For this review, take the finished solid that the model builds, in its own axes (mm). A direction names the side the tool comes from. Coordinates: 2 decimals unless noted, no trailing zeros. Write each loop counter-clockwise with the first axis right and the second up, starting at its lowest first coordinate (ties: lowest second). Pieces come first, ordered by that corner, then holes.
```python
from build123d import *

# Parameters (mm, degrees)
SKETCH8_W            = 52.5
SKETCH8_H            = 15.75
SKETCH8_R            = 0.6
SKETCH8_W_2          = 15.75
SKETCH8_H_2          = 6
BOSS_EXTRUDE13_DEPTH = 1.5


with BuildPart() as part:
    # Sketch8 → Boss-Extrude13 (new body)
    with BuildSketch(Plane.ZY):
        with Locations((-25.5, 6.625)):
            Rectangle(SKETCH8_W, SKETCH8_H)
        with Locations((-49.5, 4.75)):
            Circle(SKETCH8_R, mode=Mode.SUBTRACT)
        with Locations((-1.5, 4.75)):
            Circle(SKETCH8_R, mode=Mode.SUBTRACT)
        with Locations((-28.375, 5.75)):
            Rectangle(SKETCH8_W_2, SKETCH8_H_2, mode=Mode.SUBTRACT)
    extrude(amount=BOSS_EXTRUDE13_DEPTH)


solid = part.part
```
1) Consider section C-C (x = -0.55). Give the boundary of the cut face in (y, z).
2) The part is to be moulded in two halves that separate along Z. For faces 1 (the face through (-1, 7, -51.75)), 2 (the face through (-1, -1.25, -26)), 3 (the face through (-0.74, 4.164, -1.63)), say which applies: pulls with the +Z half, pulls with the -Z half, needs draft (parallel to the pull), parting line crosses it, or undercut.
3) Consider section B-B (y = 7.5). Give the boundary of the cut face in (x, z).
4) Clearance check with a flat-ended pin moving along its axis: P1, Ø0.7, axis at y = 4.75, z = -1.5, coming from the +X side. State where the tip first meets the part, or that it passes through.
5) Consider section A-A (z = -21.5). Give the boundary of the cut face in (x, y), then the cut area to 3 significant figures.
6) Tool access review of faces 4 (the face through (-1, 6, -20.5)), 5 (the face through (-1.5, 10, -26)): name each direction out of +Z, -Z, +X, -X, +Y, -Y from which nothing blocks a thin tool from reaching the whole face with its end or side.
7) Consider section D-D (y = 4.75). Give the boundary of the cut face in (x, z), then the cut area to 3 significant figures.
8) For L1, parallel to Y at x = -0.4, z = -49.5; L2, parallel to Z at x = -0.2, y = 6, list the stretches that pass through material, from the lowest coordinate up.
Results:
1. outline: (-1.25, -51.75) - (14.5, -51.75) - (14.5, 0.75) - (-1.25, 0.75) - close; hole (2.75, -36.25) - (8.75, -36.25) - (8.75, -20.5) - (2.75, -20.5) - close; hole circle Ø1.2 at (4.75, -49.5); hole circle Ø1.2 at (4.75, -1.5)
2. face 1: pulls with the -Z half
2. face 2: needs draft
2. face 3: undercut
3. outline: (-1.5, -51.75) - (0, -51.75) - (0, -36.25) - (-1.5, -36.25) - close; (-1.5, -20.5) - (0, -20.5) - (0, 0.75) - (-1.5, 0.75) - close
4. P1: passes through
5. outline: (-1.5, -1.25) - (0, -1.25) - (0, 2.75) - (-1.5, 2.75) - close; (-1.5, 8.75) - (0, 8.75) - (0, 14.5) - (-1.5, 14.5) - close
5. area: 14.6 mm2
6. face 4: +X, -X
6. face 5: +Z, -Z, -X, +Y, -Y
7. outline: (-1.5, -51.75) - (0, -51.75) - (0, -50.1) - (-1.5, -50.1) - close; (-1.5, -48.9) - (0, -48.9) - (0, -36.25) - (-1.5, -36.25) - close; (-1.5, -20.5) - (0, -20.5) - (0, -2.1) - (-1.5, -2.1) - close; (-1.5, -0.9) - (0, -0.9) - (0, 0.75) - (-1.5, 0.75) - close
7. area: 51.5 mm2
8. L1: y = -1.25 to 4.15, 5.35 to 14.5
8. L2: z = -51.75 to -36.25, -20.5 to 0.75
